Work out the finished part from the listing and answer in its coordinate system (mm). Give positions to 0.01 mm unless a question says otherwise; leave off trailing zeros. Loops run counter-clockwise (first coordinate to the right, second up) from the corner with the lowest first, then second, coordinate; pieces in that order, holes last. Notation, with made-up numbers: M -5,48.5 L 5,48.5 A11 ccw 5,66.5 Z; hole C 7,-11.5 d2. An arc over 180 degrees is marked long. Use a Markdown table: item, result.
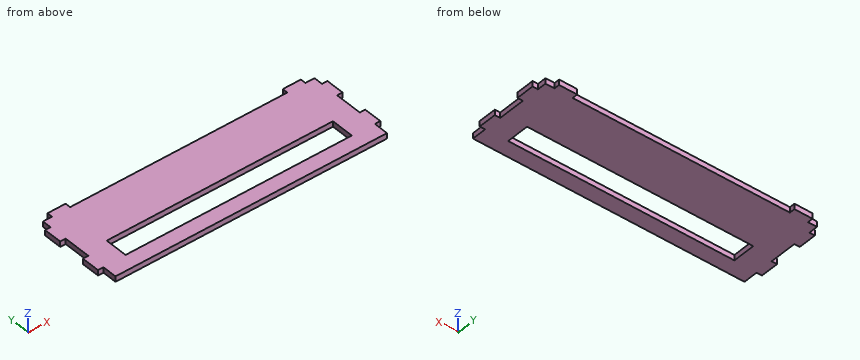
```python
from build123d import *

# Parameters (mm, degrees)
SKETCH1_W           = 250
SKETCH1_H           = 25
BOSS_EXTRUDE1_DEPTH = 6


with BuildPart() as part:
    # Sketch1 → Boss-Extrude1 (new body)
    with BuildSketch(Plane.XY):
        Polygon((495.568859933, -96.000000001), (195.568859933, -96.000000001), (195.568859933, -80.000000001), (189.568859933, -80.000000001), (189.568859933, -60.000000001), (195.568859933, -60.000000001), (195.568859933, -30.000000001), (189.568859933, -30.000000001), (189.568859933, -10.000000001), (195.568859933, -10.000000001), (195.568859933, 0), (205.568859933, 0), (205.568859933, 6), (225.568859933, 6), (225.568859933, 0), (465.568859933, 0), (465.568859933, 6), (485.568859933, 6), (485.568859933, 0), (495.568859933, 0), (495.568859933, -10), (501.568859933, -10), (501.568859933, -30), (495.568859933, -30), (495.568859933, -60), (501.568859933, -60), (501.568859933, -80), (495.568859933, -80), align=None)
        with Locations((345.568859933, -66.9)):
            Rectangle(SKETCH1_W, SKETCH1_H, mode=Mode.SUBTRACT)
    extrude(amount=-BOSS_EXTRUDE1_DEPTH)


solid = part.part
```
(1) Consider probe 1 along X at (y, z) = (-76, -4.65); probe 2 along Y at (x, z) = (464.5, -1.3); probe 3 along X at (y, z) = (1.5, -0.75). Determine where each line is inside the solid, lowest interval first. Write a range as [from, to].
Entries:
| item | result |
|---|---|
| probe 1 | x = [189.57, 220.57], [470.57, 501.57] |
| probe 2 | y = [-96, -79.4], [-54.4, 0] |
| probe 3 | x = [205.57, 225.57], [465.57, 485.57] |
(2) A cutting plane is placed at A-A (x = 359). Write down the section's boundary in (y, z), and give its area (3 significant figures).
Entries:
| item | result |
|---|---|
| outline | M -96,-6 L -79.4,-6 L -79.4,0 L -96,0 Z; M -54.4,-6 L 0,-6 L 0,0 L -54.4,0 Z |
| area | 426 mm² |
(3) A cutting plane is placed at C-C (y = -5). Write down the section's boundary in (x, z).
Entries:
| item | result |
|---|---|
| outline | M 195.57,-6 L 495.57,-6 L 495.57,0 L 195.57,0 Z |
(4) Given P1, Ø3, axis at x = 191.5, z = -2, coming from the +Y side; P2, Ø1.8, axis at x = 191, z = -3.5, coming from the -Y side; P3, Ø1.8, axis at x = 395.5, z = -4, coming from the +Y side, each flat-ended and moving along its own axis, determine where each tip first touches the part or whether it passes through.
Entries:
| item | result |
|---|---|
| P1 | stops at y = -10 |
| P2 | stops at y = -80 |
| P3 | stops at y = 0 |
